Read the model definition and answer for the solid it produces. Units are mm, in the model's axes. Face numbers are marked on the shaded views. Give positions to 0.01 mm unless a question says otherwise; leave off trailing zeros. Loops run counter-clockwise (first coordinate to the right, second up) from the corner with the lowest first, then second, coordinate; pieces in that order, holes last. Notation, with made-up numbers: (64, 89.25) - (90, 89.25) arc R25 ccw to (90, 122.25) - close; hole circle Ø4 at (-5.75, 52.5). An arc over 180 degrees is marked (long way). Put each result on its own line as item: value. Start each with the question number.
1. For a pull along Y with two mould halves and no side action, classify the marked faces 1, 2 and 3 as released by +Y, released by -Y, zero draft, split by the parting line, or undercut.
2. A cutting plane is placed at A-A, the plane x = 0. Determine the outline of the cut face in (y, z).
3. Consider L1, parallel to Y at x = 0, z = 86.25; L2, parallel to Z at x = -3, y = 6.5; L3, parallel to Z at x = -17, y = 18. Determine where each line is inside the solid, lowest interval first. Write a range as from..to.
4. A cutting plane is placed at C-C, the plane z = 66. Determine the outline of the cut face in (x, y).
5. Given pin 1 Ø22 at (x, y) = (5.5, 6) entering from +Z; pin 2 Ø4 at (y, z) = (-23.5, 66.5) entering from -X; pin 3 Ø6.5 at (x, z) = (-24.5, 96) entering from +Y, each flat-ended and moving along its own axis, determine where each tip first touches the part or whether it passes through.
6. A cutting plane is placed at D-D, the plane x = -20. Determine the outline of the cut face in (y, z).
```python
from build123d import *

# Parameters (mm, degrees)
CYLINDER001_R     = 22
CYLINDER001_DEPTH = 20
BOX_W             = 20
BOX_H             = 10
BOX_DEPTH         = 10
ARRAY_COUNT       = 8
CYLINDER_R        = 30
CYLINDER_DEPTH    = 100


with BuildPart() as cilindre001:
    # Cylinder001 → Cylinder001 (new body)
    with BuildSketch(Plane.XY.offset(80)):
        Circle(CYLINDER001_R)
    extrude(amount=CYLINDER001_DEPTH)


with BuildPart() as array:
    # Box → Box (new body)
    with BuildSketch(Plane(origin=(18, -5, 0), x_dir=(1, 0, 0), z_dir=(0, 0, 1))):
        with Locations((10, 5)):
            Rectangle(BOX_W, BOX_H)
    extrude(amount=BOX_DEPTH)

    # Array: Array ×8 about axis
    array_axis = Axis((0, 0, 0), (0, 0, 1))


with BuildPart() as array_1:
    add(array.part)
    for i in range(1, ARRAY_COUNT):
        add(array.part.rotate(array_axis, i * 360 / ARRAY_COUNT))


with BuildPart() as array_2:
    # Array placement: moved
    add(array_1.part.moved(Location((0, 0, 92))))


with BuildPart() as cut001:
    # Cylinder → Cylinder (new body)
    with BuildSketch(Plane.XY):
        Circle(CYLINDER_R)
    extrude(amount=CYLINDER_DEPTH)

    # Cut: cut Array
    add(array_2.part, mode=Mode.SUBTRACT)

    # Cut001: cut Cilindre001
    add(cilindre001.part, mode=Mode.SUBTRACT)


solid = cut001.part
```
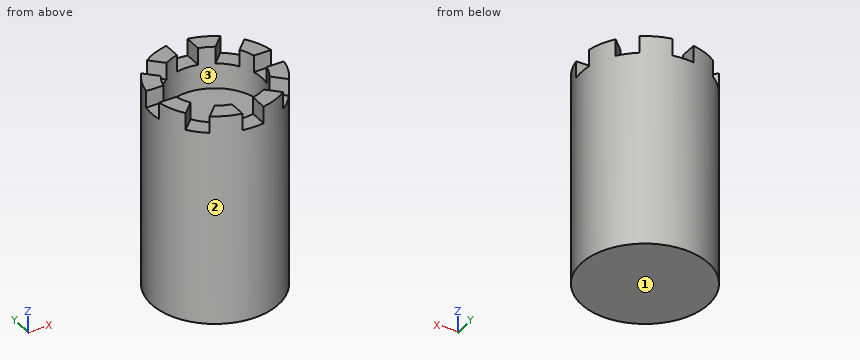
Return value:
1. face 1: zero draft
1. face 2: split by the parting line
1. face 3: undercut
2. outline: (-30, 0) - (30, 0) - (30, 92) - (22, 92) - (22, 80) - (-22, 80) - (-22, 92) - (-30, 92) - close
3. L1: y = -30..-22, 22..30
3. L2: z = 0..80
3. L3: z = 0..92
4. outline: circle Ø60 at (0, 0)
5. pin 1: stops at z = 80
5. pin 2: stops at x = -20.92
5. pin 3: stops at y = 17.38
6. outline: (-22.36, 0) - (22.36, 0) - (22.36, 92) - (12.93, 92) - (12.93, 100) - (9.17, 100) - (9.17, 80) - (-9.17, 80) - (-9.17, 100) - (-12.93, 100) - (-12.93, 92) - (-22.36, 92) - close
